The listing builds one solid part. Answer for the finished solid, in the listing's coordinates (mm). Face numbers are marked on the shaded views. A direction names the side the tool comes from. Coordinates: 2 decimals unless noted, no trailing zeros. Write each loop counter-clockwise with the first axis right and the second up, starting at its lowest first coordinate (ties: lowest second). Pieces come first, ordered by that corner, then holes.
from build123d import *

# Parameters (mm, degrees)
SKETCH1_R           = 41.25
BOSS_EXTRUDE1_DEPTH = 15
SKETCH2_R           = 31.75
CUT_EXTRUDE1_DEPTH  = 0.508
SKETCH3_R           = 29.21
CUT_EXTRUDE2_DEPTH  = 2.032
CUT_EXTRUDE2_TAPER  = 60
SKETCH4_R           = 8.89
BOSS_EXTRUDE3_DEPTH = 1.016
BOSS_EXTRUDE3_TAPER = 30
SKETCH5_RX          = 5.334
SKETCH5_RY          = 3.81
CUT_EXTRUDE3_DEPTH  = 13.46
CIRPATTERN1_COUNT   = 8
SKETCH6_R           = 35.408
CUT_EXTRUDE4_DEPTH  = 2.286


with BuildPart() as part:
    # Sketch1 → Boss-Extrude1 (new body)
    with BuildSketch(Plane(origin=(0, 0, 0), x_dir=(0, 0, -1), z_dir=(1, 0, 0))):
        Circle(SKETCH1_R)
    extrude(amount=BOSS_EXTRUDE1_DEPTH)

    # Sketch2 → Cut-Extrude1 (cut)
    with BuildSketch(Plane(origin=(15, 0, 0), x_dir=(0, 0, -1), z_dir=(1, 0, 0))):
        Circle(SKETCH2_R)
    extrude(amount=-CUT_EXTRUDE1_DEPTH, mode=Mode.SUBTRACT)

    # Sketch3 → Cut-Extrude2 (cut)
    with BuildSketch(Plane(origin=(14.492, 0, 0), x_dir=(0, 0, -1), z_dir=(1, 0, 0))):
        Circle(SKETCH3_R)
    extrude(amount=-CUT_EXTRUDE2_DEPTH, taper=CUT_EXTRUDE2_TAPER, mode=Mode.SUBTRACT)

    # Sketch4 → Boss-Extrude3 (add)
    with BuildSketch(Plane(origin=(12.46, 0, 0), x_dir=(0, 0, -1), z_dir=(1, 0, 0))):
        Circle(SKETCH4_R)
    extrude(amount=BOSS_EXTRUDE3_DEPTH, taper=BOSS_EXTRUDE3_TAPER)

    # Sketch5 → Cut-Extrude3 (cut, through all)
    with BuildSketch(Plane(origin=(12.46, 0, 0), x_dir=(0, 0, -1), z_dir=(1, 0, 0))):
        with Locations(Location((0.079644617, 16.836924445), (0, 0, -90))):
            Ellipse(SKETCH5_RX, SKETCH5_RY)
    cut_extrude3 = extrude(amount=-CUT_EXTRUDE3_DEPTH, mode=Mode.SUBTRACT)

    # CirPattern1: Cut-Extrude3 ×8 about axis
    cirpattern1_axis = Axis((13.476, 0, 0), (1, 0, 0))
    for i in range(1, CIRPATTERN1_COUNT):
        add(cut_extrude3.rotate(cirpattern1_axis, i * 360 / CIRPATTERN1_COUNT), mode=Mode.SUBTRACT)

    # Sketch6 → Cut-Extrude4 (cut)
    with BuildSketch(Plane.ZY):
        Circle(SKETCH6_R)
    extrude(amount=-CUT_EXTRUDE4_DEPTH, mode=Mode.SUBTRACT)

    # Sketch7 → Cut-Revolve1 (revolve, cut)
    with BuildSketch(Plane.XY):
        with BuildLine():
            Line((7.5, 41.25), (0, 41.25))
            Line((0, 41.25), (0, 37.82380131))
            ThreePointArc((0, 37.82380131), (7.5, 41.240433802), (15, 37.82380131))
            Line((15, 37.82380131), (15, 41.25))
            Line((15, 41.25), (7.5, 41.25))
        make_face()
    revolve(axis=Axis((0, 0, 0), (1, 0, 0)), mode=Mode.SUBTRACT)


solid = part.part
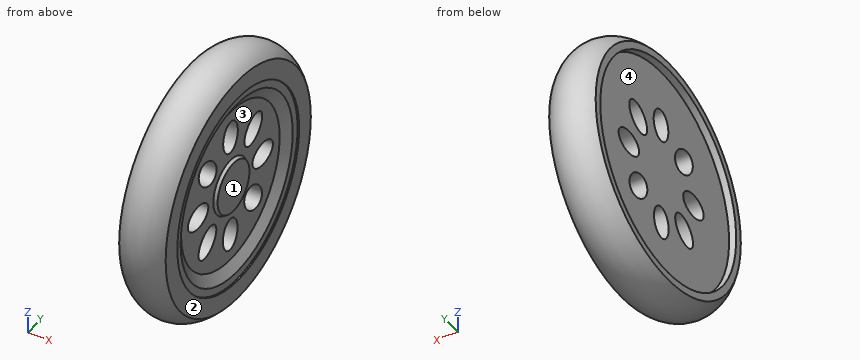
Q1. The part is cut by section B-B, the plane x = 8. State how many separate pieces and enclosed holes the cut face has, then the cut area to 3 significant figures.
Answers below:
separate pieces: 1
enclosed holes: 8
area: 4,830 mm2
Q2. Find the intervals of material crossed by probe 1 along Y at (x, z) = (4.25, -3); probe 2 along Y at (x, z) = (8.5, 10.5); probe 3 along Z at (x, y) = (8.5, -13), in increasing order.
Answers below:
probe 1: y = -40.58 to -19.98, -13.7 to 13.41, 20.26 to 40.58
probe 2: y = -39.83 to -15.54, -7.21 to 7.33, 15.72 to 39.83
probe 3: z = -39.08 to -16.46, -7.91 to -2.57, 2.73 to 8.09, 16.58 to 39.08
Q3. Given pin 1 (2 mm diameter, centred on x = 7.5, z = -2, fed in from -Y); pin 2 (4 mm diameter, centred on x = 5, y = 31.5, fed in from +Z); pin 3 (3 mm diameter, centred on y = 12, z = 12.5, fed in from -X); pin 4 (1.5 mm diameter, centred on x = 4.5, z = 10, fed in from -Y), each flat-ended and moving along its own axis, determine where each tip first touches the part or whether it passes through.
Answers below:
pin 1: stops at y = -41.23
pin 2: stops at z = 28.46
pin 3: passes through
pin 4: stops at y = -39.82
Q4. The part is cut by section A-A, the plane x = 1.25. Write down the section's boundary in (y, z), then the cut area to 3 significant figures.
Answers below:
outline: circle Ø78.06 at (0, 0); hole circle Ø70.82 at (0, 0)
area: 847 mm2
Q5. Determine the mould class of the marked faces 1 and 2 for opening direction Z: released by +Z, released by -Z, zero draft, split by the parting line, or undercut.
Answers below:
face 1: undercut
face 2: zero draft
Q6. Which of the six approach directions +Z, -Z, +X, -X, +Y, -Y give full straight-line access (tool end or side, diameter ignored) to the marked faces 3 and 4?
Answers below:
face 3: +X
face 4: -X
